```python
from build123d import *

# Parameters (mm, degrees)
DODANIE_WYCI_GNI_CIE1_DEPTH = 5
SZKIC2_R                    = 6.235949903
DODANIE_WYCI_GNI_CIE2_DEPTH = 1


with BuildPart() as part:
    # Szkic1 → Dodanie-wyciągnięcie1 (new body)
    with BuildSketch(Plane(origin=(0, 0, 0), x_dir=(0, 0, -1), z_dir=(1, 0, 0))):
        with BuildLine():
            Line((16.683684026, -85.628014752), (41.227039969, -76.881944554))
            ThreePointArc((41.227039969, -76.881944554), (46.201703182, -59.964643396), (63.82826816, -59.468095705))
            Line((63.82826816, -59.468095705), (78.543449139, -37.966153615))
            ThreePointArc((78.543449139, -37.966153615), (72.624296091, -21.355735808), (86.5926233, -10.593385344))
            Line((86.5926233, -10.593385344), (85.858930332, 15.451417583))
            ThreePointArc((85.858930332, 15.451417583), (71.306876302, 25.410337004), (76.281539514, 42.327638162))
            Line((76.281539514, 42.327638162), (60.379218375, 62.967072438))
            ThreePointArc((60.379218375, 62.967072438), (42.752653397, 62.470524746), (36.833500348, 79.080942553))
            Line((36.833500348, 79.080942553), (11.836697213, 86.431445794))
            ThreePointArc((11.836697213, 86.431445794), (-2.131629996, 75.669095331), (-16.683684026, 85.628014752))
            Line((-16.683684026, 85.628014752), (-41.227039969, 76.881944554))
            ThreePointArc((-41.227039969, 76.881944554), (-46.201703182, 59.964643396), (-63.82826816, 59.468095705))
            Line((-63.82826816, 59.468095705), (-78.543449139, 37.966153615))
            ThreePointArc((-78.543449139, 37.966153615), (-72.624296091, 21.355735808), (-86.5926233, 10.593385344))
            Line((-86.5926233, 10.593385344), (-85.858930332, -15.451417583))
            ThreePointArc((-85.858930332, -15.451417583), (-71.306876302, -25.410337004), (-76.281539514, -42.327638162))
            Line((-76.281539514, -42.327638162), (-60.379218375, -62.967072438))
            ThreePointArc((-60.379218375, -62.967072438), (-42.752653397, -62.470524746), (-36.833500348, -79.080942553))
            Line((-36.833500348, -79.080942553), (-11.836697213, -86.431445794))
            ThreePointArc((-11.836697213, -86.431445794), (2.131629996, -75.669095331), (16.683684026, -85.628014752))
        make_face()
    extrude(amount=DODANIE_WYCI_GNI_CIE1_DEPTH)

    # Szkic2 → Dodanie-wyciągnięcie2 (add)
    with BuildSketch(Plane(origin=(5, 0, 0), x_dir=(0, 0, -1), z_dir=(1, 0, 0))):
        Circle(SZKIC2_R)
    extrude(amount=DODANIE_WYCI_GNI_CIE2_DEPTH)


solid = part.part
```
Could you check a few things on this model? Use its own coordinates, in mm. Round coordinates to 2 decimals unless told otherwise and drop trailing zeros. Loops run counter-clockwise (first coordinate to the right, second up) from the corner with the lowest first, then second, coordinate; pieces in that order, holes last.
Q1. For P1, Ø4, axis at y = 3, z = 18, coming from the +X side; P2, Ø1, axis at x = 2.5, z = -47, coming from the -Y side, each with a flat end and sliding along its axis, tell me the tip position at first contact or that it passes through.
Q2. I want a section at D-D (z = -45.5). Write out the boundary of the cut face in (x, y), and give its area (3 significant figures).
Q3. Thinking about a two-plate mould opening in Y: for faces 1 (the cylindrical face through (2.46, 21.61, 72.55)), 2 (the flat face through (2.465, -81.316, -28.784)), 3 (the flat face through (2.465, 82.705, -24.51)), 4 (the cylindrical face through (2.465, -62.323, 42.972)), which applies, pulls with the +Y half, pulls with the -Y half, needs draft (parallel to the pull), parting line crosses it, or undercut?
Q4. I want a section at B-B (z = -4). Write out the boundary of the cut face in (x, y), and give its area (3 significant figures).
Q5. Please list where these lines run through material, in increasing order: L1, parallel to X at y = -54.5, z = 25; L2, parallel to Y at x = 2, z = -26.5; L3, parallel to Y at x = 1.1, z = -22.
Q6. I want a section at C-C (y = -4). Write out the boundary of the cut face in (x, z).
Q7. I want a section at A-A (x = 1.35). Write out the boundary of the cut face in (y, z), and give its area (3 significant figures).
Answer below:
1. P1: stops at x = 5
1. P2: stops at y = -59.74
2. outline: (0, -60.54) - (5, -60.54) - (5, 60.98) - (0, 60.98) - close
2. area: 608 mm2
3. face 1: undercut
3. face 2: pulls with the -Y half
3. face 3: pulls with the +Y half
3. face 4: undercut
4. outline: (0, -75.73) - (5, -75.73) - (5, -4.78) - (6, -4.78) - (6, 4.78) - (5, 4.78) - (5, 77.17) - (0, 77.17) - close
4. area: 774 mm2
5. L1: x = 0 to 5
5. L2: y = -82.13 to 82.12
5. L3: y = -83.73 to 83.44
6. outline: (0, -86.41) - (5, -86.41) - (5, -4.78) - (6, -4.78) - (6, 4.78) - (5, 4.78) - (5, 86.18) - (0, 86.18) - close
7. outline: (-86.43, 11.84) arc R15 cw to (-85.63, -16.68) - (-76.88, -41.23) arc R15 cw to (-59.47, -63.83) - (-37.97, -78.54) arc R15 cw to (-10.59, -86.59) - (15.45, -85.86) arc R15 cw to (42.33, -76.28) - (62.97, -60.38) arc R15 cw to (79.08, -36.83) - (86.43, -11.84) arc R15 cw to (85.63, 16.68) - (76.88, 41.23) arc R15 cw to (59.47, 63.83) - (37.97, 78.54) arc R15 cw to (10.59, 86.59) - (-15.45, 85.86) arc R15 cw to (-42.33, 76.28) - (-62.97, 60.38) arc R15 cw to (-79.08, 36.83) - close
7. area: 21,300 mm2
